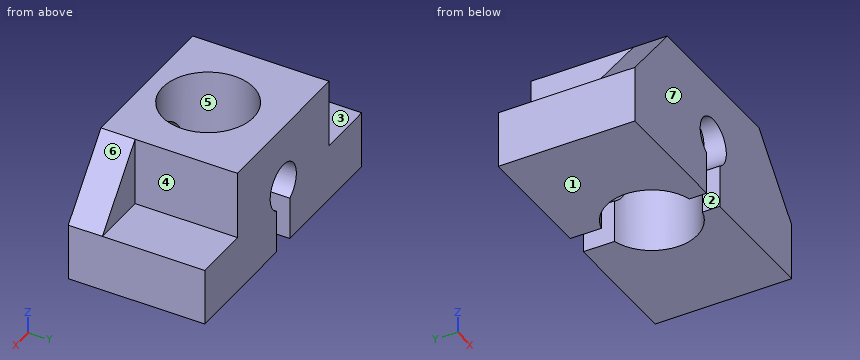
```python
from build123d import *

# Parameters (mm, degrees)
F2_DEPTH  = 600
F3_W      = 250
F3_H      = 300
F4_DEPTH  = 600
F6_DEPTH  = 150
F8_DEPTH  = 150
F9_R      = 200
F10_DEPTH = 550.001


with BuildPart() as f2:
    # F1 (on face) → F2 (new body)
    with BuildSketch(Plane.XZ):
        with BuildLine():
            Line((600, -275), (600, 275))
            Line((600, 275), (-600, 275))
            Line((-600, 275), (-600, -275))
            Line((-600, -275), (-50, -275))
            Line((-50, -275), (-50, -86.6025403784))
            ThreePointArc((-50, -86.6025403784), (0, 100), (50, -86.6025403784))
            Line((50, -86.6025403784), (50, -100))
            Line((50, -100), (50, -101.5080809593))
            Line((50, -101.5080809593), (50, -275))
            Line((50, -275), (600, -275))
        make_face()
    extrude(amount=F2_DEPTH)

    # F3 (on face) → F4 (cut)
    with BuildSketch(Plane.XZ.offset(600)):
        with Locations((-475, 125)):
            Rectangle(F3_W, F3_H)
        with Locations((475, 125)):
            Rectangle(F3_W, F3_H)
    extrude(amount=-F4_DEPTH, mode=Mode.SUBTRACT)

    # F5 (on face) → F6 (join)
    with BuildSketch(Plane.XZ.offset(600)):
        Polygon((-350, 275), (-600, -25), (-350, -25), align=None)
    extrude(amount=-F6_DEPTH)

    # F7 (on face) → F8 (join)
    with BuildSketch(Plane.XZ.offset(600)):
        Polygon((350, -25), (600, -25), (350, 275), align=None)
    extrude(amount=-F8_DEPTH)

    # F9 (on face) → F10 (cut, through all)
    with BuildSketch(Plane.XY.offset(275)):
        with Locations((0, -330.283343792)):
            Circle(F9_R)
    extrude(amount=-F10_DEPTH, mode=Mode.SUBTRACT)


solid = f2.part
```
Part model, mm, in its own coordinate system. Face numbers are marked on the shaded views. A direction names the side the tool comes from. Round coordinates to 2 decimals unless told otherwise and drop trailing zeros. Loops run counter-clockwise (first coordinate to the right, second up) from the corner with the lowest first, then second, coordinate; pieces in that order, holes last. Notation, with made-up numbers: (74.25, 13.5) -> (84.25, 13.5) arc R20 cw to (84.25, 17.5) -> close; hole circle Ø3 at (33, 0.5). An arc over 180 degrees is marked (long way). Use CSV: the item, a comma, the result in double quotes. Start each with the question number.
1) Which spindle directions (+Z, -Z, +X, -X, +Y, -Y) get a long thin tool onto all of the face, cutting with end or side? Do the marked faces 1, 2, 3 and 4. Say none if no direction does.
2) Cut at D-D, the plane y = -85.5. Write the cut outline in (x, z), plus the area to 3 significant figures.
3) Pull direction Y, two halves, no side cores. Call the marked faces 5, 6 and 7: +Y half, -Y half, draft (parallel to the pull), parting line (faces both ways), or undercut.
4) Wall check: L1, parallel to Z at x = -388, y = -265; L2, parallel to X at y = -92, z = 0; L3, parallel to X at y = -328, z = 48.5. Give the ranges that are in metal, low to high. Write a range as [from, to].
5) Drop a flat-ended pin along its axis: P1, Ø8, axis at y = -75.5, z = 122, coming from the +X side. Give the stop position or say it passes through.
6) Cut at C-C, the plane z = 46. Write the cut outline in (x, y), plus the area to 3 significant figures.
7) Cut at A-A, the plane x = 0. Write the cut outline in (y, z), plus the area to 3 significant figures.
8) Cut at B-B, the plane y = -487. Write the cut outline in (x, z), plus the area to 3 significant figures.
Determined:
1,face 1,"-Z, +X, -X, +Y, -Y"
1,face 2,"-Z, +Y, -Y"
1,face 3,"+Z, -X, +Y"
1,face 4,"+Z, +X, +Y"
2,outline,"(-600, -275) -> (-50, -275) -> (-50, -86.6) arc R100 cw (long way) to (50, -86.6) -> (50, -275) -> (600, -275) -> (600, -25) -> (350, -25) -> (350, 275) -> (-350, 275) -> (-350, -25) -> (-600, -25) -> close"
2,area,"461,000 mm2"
3,face 5,"undercut"
3,face 6,"draft"
3,face 7,"-Y half"
4,L1,"z = [-275, -25]"
4,L2,"x = [-350, -100], [100, 350]"
4,L3,"x = [-350, -199.99], [199.99, 350]"
5,P1,"stops at x = 350"
6,outline,"(-540.83, -600) -> (-88.79, -600) -> (-88.79, -509.49) arc R200 cw to (-88.79, -151.07) -> (-88.79, 0) -> (-350, 0) -> (-350, -450) -> (-540.83, -450) -> close; (88.79, -600) -> (540.83, -600) -> (540.83, -450) -> (350, -450) -> (350, 0) -> (88.79, 0) -> (88.79, -151.07) arc R200 cw to (88.79, -509.49) -> close"
6,area,"314,000 mm2"
7,outline,"(-600, 100) -> (-530.28, 100) -> (-530.28, 275) -> (-600, 275) -> close; (-130.28, 100) -> (0, 100) -> (0, 275) -> (-130.28, 275) -> close"
7,area,"35,000 mm2"
8,outline,"(-600, -275) -> (-124.26, -275) -> (-124.26, 275) -> (-350, 275) -> (-600, -25) -> close; (124.26, -275) -> (600, -275) -> (600, -25) -> (350, 275) -> (124.26, 275) -> close"
8,area,"448,000 mm2"
